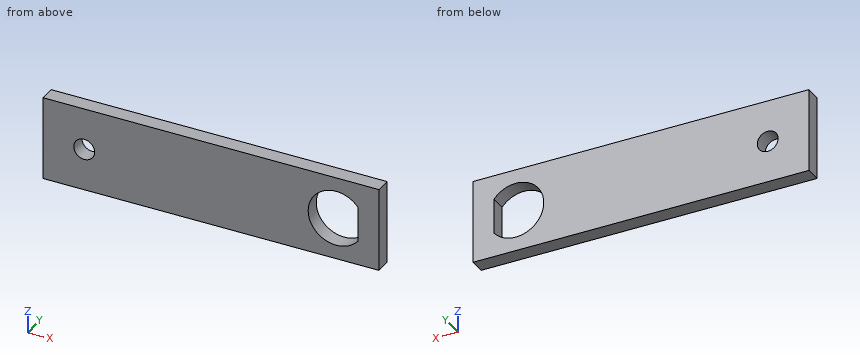
from build123d import *

# Parameters (mm, degrees)
SKETCH1_W           = 76.2
SKETCH1_H           = 19.05
SKETCH1_R           = 2.37
BOSS_EXTRUDE1_DEPTH = 3.5


with BuildPart() as part:
    # Sketch1 → Boss-Extrude1 (new body)
    with BuildSketch(Plane(origin=(0, 0, 0), x_dir=(1, 0, 0), z_dir=(0, 1, 0))):
        with Locations((38.1, 9.525)):
            Rectangle(SKETCH1_W, SKETCH1_H)
        with Locations((9.35, 9.525)):
            Circle(SKETCH1_R, mode=Mode.SUBTRACT)
        with BuildLine():
            Line((71.433, 13.523501094), (71.433, 5.526498906))
            ThreePointArc((71.433, 5.526498906), (60.15, 9.525), (71.433, 13.523501094))
        make_face(mode=Mode.SUBTRACT)
    extrude(amount=BOSS_EXTRUDE1_DEPTH)


solid = part.part
Can you work these out from the model? Positions are in its coordinate system, mm. Round coordinates to 2 decimals unless told otherwise and drop trailing zeros. Write each loop counter-clockwise with the first axis right and the second up, starting at its lowest first coordinate (ties: lowest second). Pieces come first, ordered by that corner, then holes. Notation, with made-up numbers: (21.5, -9) -> (33.5, -9) arc R12 ccw to (33.5, -1) -> close; hole circle Ø8 at (-16.5, -8.75). An arc over 180 degrees is marked (long way). Use one line per item in the form item = value. Start each with the question number.
Q1. Imagine slicing it at D-D (z = -11.25). Please give me the cut outline in (x, y).
Q2. I'm going to push a flat-ended pin straight in: P1, Ø4, axis at x = 9.35, z = -9.525, coming from the -Y side. Where does the tip first touch, or does it pass through?
Q3. Imagine slicing it at C-C (y = 0.8). Count the separate pieces of the cut face and the enclosed holes in it, then the cut area to 3 significant figures.
Q4. Imagine slicing it at A-A (x = 9.35). Please give me the cut outline in (y, z) (3 decimals), then the cut area to 3 significant figures.
Q5. Imagine slicing it at B-B (z = -4). Please give me the cut outline in (x, y).
Q6. If I drill on probe 1 along Z at (x, y) = (66.5, 1.45) (3 decimals); probe 2 along Z at (x, y) = (9.35, 1.55) (3 decimals); probe 3 along X at (y, z) = (1.8, -10.75), over which ranges is the centre line in solid material (lowest first)? Write a range as [from, to].
Worked out:
q1.outline = (0, 0) -> (7.72, 0) -> (7.72, 3.5) -> (0, 3.5) -> close; (10.98, 0) -> (60.39, 0) -> (60.39, 3.5) -> (10.98, 3.5) -> close; (71.43, 0) -> (76.2, 0) -> (76.2, 3.5) -> (71.43, 3.5) -> close
q2.P1 = through
q3.separate_pieces = 1
q3.enclosed_holes = 2
q3.area = 1,320 mm^2
q4.outline = (0, -19.05) -> (3.5, -19.05) -> (3.5, -11.895) -> (0, -11.895) -> close; (0, -7.155) -> (3.5, -7.155) -> (3.5, 0) -> (0, 0) -> close
q4.area = 50.1 mm^2
q5.outline = (0, 0) -> (63.37, 0) -> (63.37, 3.5) -> (0, 3.5) -> close; (69.63, 0) -> (76.2, 0) -> (76.2, 3.5) -> (69.63, 3.5) -> close
q6.probe_1 = [-19.05, -15.875], [-3.175, 0]
q6.probe_2 = [-19.05, -11.895], [-7.155, 0]
q6.probe_3 = [0, 7.32], [11.38, 60.27], [71.43, 76.2]
